Work out the finished part from the listing and answer in its coordinate system (mm). A direction names the side the tool comes from. Give positions to 0.01 mm unless a question says otherwise; leave off trailing zeros. Loops run counter-clockwise (first coordinate to the right, second up) from the corner with the lowest first, then second, coordinate; pieces in that order, holes last. Notation, with made-up numbers: M 53.5,0 L 84.5,0 A8 ccw 84.5,5 Z; hole C 57.25,49.25 d2. An arc over 180 degrees is marked long. Answer as a JSON object with one key per item and string values. Group by question number.
Autodesk Inventor part; units mm, degrees
ref_plane "YZ Plane" through (0, 0, 0) normal (1, 0, 0) x (0, 1, 0)
ref_plane "XZ Plane" through (0, 0, 0) normal (0, 1, 0) x (-1, 0, 0)
ref_plane "XY Plane" through (0, 0, 0) normal (0, 0, 1) x (1, 0, 0)
sketch "Sketch1" plane through (0, 0, 0) normal (0, 0, 1) x (1, 0, 0)
  line L0 (0, 0) -> (57.15, 0)
  line L1 (57.15, 0) -> (57.15, 25.4)
  line L2 (57.15, 25.4) -> (0, 25.4)
  line L3 (0, 25.4) -> (0, 0)
  dimension "d0" = 57.15
  dimension "d1" = 25.4
extrude "Extrusion1" add sketch "Sketch1" along normal blind 38.1
sketch "Sketch2" plane through (0, 0, 38.1) normal (0, 0, 1) x (1, 0, 0)
  point P0 (0, 0)
sketch "Sketch3" plane through (0, 0, 38.1) normal (0, 0, 1) x (1, 0, 0)
  line L0 (57.355, 0) -> (57.15, 12.7)
  line L1 (57.15, 0) -> (57.15, 25.4)
  line L2 (57.15, 12.7) -> (12.7, 12.7)
  line L3 (12.7, 12.7) -> (12.7, 0)
  line L4 (0, 0) -> (57.15, 0)
  line L5 (57.15, 0) -> (12.7, 0)
  dimension "d4" = 44.45
extrude "Extrusion2" cut sketch "Sketch3" against normal blind 38.1
draft "FaceDraft1" angle 35 pull direction (0, 0, 1) faces at (12.7, 8.4667, 25.4) fixed edges at (12.7, 6.35, 38.1)
chamfer "Chamfer1" distance 19.05 angle 45 1 edges at (57.15, 19.05, 38.1)
properties part number "Unit 7.1 part 4"
Item 1: Find the intervals of material crossed by probe 1 along Y at (x, z) = (40, 33); probe 2 along X at (y, z) = (11.25, 24); probe 3 along Z at (x, y) = (16.5, 2), in increasing order. Write a range as [from, to].
Item 2: A cutting plane is placed at B-B (z = 35). Determine the outline of the cut face in (x, y), and give its area (3 significant figures).
Item 3: A tool of negligible diameter and unlimited length cuts with its end or side. For faces 1 (the flat face through (40, 12.7, 19)), 2 (the flat face through (0, 13, 19)), from which of +Z, -Z, +X, -X, +Y, -Y can it reach the whole face along a straight path? Write none if from no direction.
Item 4: A cutting plane is placed at C-C (x = 48). Determine the outline of the cut face in (y, z), and give its area (3 significant figures).
Item 5: A cutting plane is placed at D-D (y = 9.25). Determine the outline of the cut face in (x, z), and give its area (3 significant figures).
Item 6: Given pin 1 Ø5 at (x, z) = (49.5, 31) entering from +Y, flat-ended and moving along its own axis, determine where the tip first touches the part or whether it passes through.
Item 7: A cutting plane is placed at A-A (y = 20.25). Determine the outline of the cut face in (x, z), and give its area (3 significant figures).
The answers:
{
 "1": {"probe 1": "y = [12.7, 25.4]", "probe 2": "x = [0, 22.57]", "probe 3": "z = [0, 32.67]"},
 "2": {"outline": "M 0,0 L 14.87,0 L 14.87,12.7 L 41.2,12.7 L 41.2,25.4 L 0,25.4 Z", "area": "712 mm^2"},
 "3": {"face 1": "+Z, +X, -Y", "face 2": "+Z, -Z, -X, +Y, -Y"},
 "4": {"outline": "M 12.7,0 L 25.4,0 L 25.4,28.2 L 12.7,28.2 Z", "area": "358 mm^2"},
 "5": {"outline": "M 0,0 L 39.38,0 L 12.7,38.1 L 0,38.1 Z", "area": "992 mm^2"},
 "6": {"pin 1": "passes through"},
 "7": {"outline": "M 0,0 L 57.15,0 L 57.15,19.05 L 38.1,38.1 L 0,38.1 Z", "area": "2,000 mm^2"}
}
